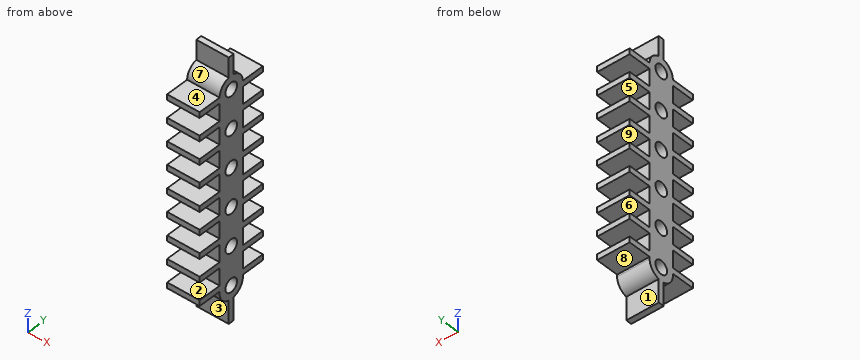
```python
from build123d import *

# Parameters (mm, degrees)
SKETCH1_R           = 17.5
BOSS_EXTRUDE1_DEPTH = 85


with BuildPart() as part:
    # Sketch1 → Boss-Extrude1 (new body)
    with BuildSketch(Plane(origin=(0, 0, 0), x_dir=(0, 0, -1), z_dir=(1, 0, 0))):
        with BuildLine():
            Line((-250.081967213, 35), (-205.081967213, 35))
            Line((-205.081967213, 35), (-205.081967213, 95))
            Line((-205.081967213, 95), (-190.081967213, 95))
            Line((-190.081967213, 95), (-190.081967213, 35))
            Line((-190.081967213, 35), (-185.081967213, 35))
            Line((-185.081967213, 35), (-145.081967213, 35))
            Line((-145.081967213, 35), (-145.081967213, 95))
            Line((-145.081967213, 95), (-130.081967213, 95))
            Line((-130.081967213, 95), (-130.081967213, 35))
            Line((-130.081967213, 35), (-85.081967213, 35))
            Line((-85.081967213, 35), (-85.081967213, 95))
            Line((-85.081967213, 95), (-70.081967213, 95))
            Line((-70.081967213, 95), (-70.081967213, 35))
            Line((-70.081967213, 35), (-25.081967213, 35))
            Line((-25.081967213, 35), (-25.081967213, 95))
            Line((-25.081967213, 95), (-10.081967213, 95))
            Line((-10.081967213, 95), (-10.081967213, 35))
            Line((-10.081967213, 35), (34.918032787, 35))
            Line((34.918032787, 35), (34.918032787, 95))
            Line((34.918032787, 95), (49.918032787, 95))
            Line((49.918032787, 95), (49.918032787, 35))
            Line((49.918032787, 35), (94.918032787, 35))
            Line((94.918032787, 35), (94.918032787, 95))
            Line((94.918032787, 95), (109.918032787, 95))
            Line((109.918032787, 95), (109.918032787, 35))
            Line((109.918032787, 35), (154.918032787, 35))
            Line((154.918032787, 35), (154.918032787, 95))
            Line((154.918032787, 95), (169.918032787, 95))
            Line((169.918032787, 95), (169.918032787, 35))
            Line((169.918032787, 35), (214.918032787, 35))
            Line((214.918032787, 35), (214.918032787, 95))
            Line((214.918032787, 95), (229.918032787, 95))
            Line((229.918032787, 95), (229.918032787, 35))
            Line((229.918032787, 35), (235.374517149, 35))
            ThreePointArc((235.374517149, 35), (257.311928117, 27.271780287), (269.561502977, 7.5))
            Line((269.561502977, 7.5), (329.561502977, 7.5))
            Line((329.561502977, 7.5), (329.561502977, -7.5))
            Line((329.561502977, -7.5), (269.561502977, -7.5))
            ThreePointArc((269.561502977, -7.5), (257.311928117, -27.271780287), (235.374517149, -35))
            Line((235.374517149, -35), (229.918032787, -35))
            Line((229.918032787, -35), (229.918032787, -95))
            Line((229.918032787, -95), (214.918032787, -95))
            Line((214.918032787, -95), (214.918032787, -35))
            Line((214.918032787, -35), (169.918032787, -35))
            Line((169.918032787, -35), (169.918032787, -95))
            Line((169.918032787, -95), (154.918032787, -95))
            Line((154.918032787, -95), (154.918032787, -35))
            Line((154.918032787, -35), (109.918032787, -35))
            Line((109.918032787, -35), (109.918032787, -95))
            Line((109.918032787, -95), (94.918032787, -95))
            Line((94.918032787, -95), (94.918032787, -35))
            Line((94.918032787, -35), (49.918032787, -35))
            Line((49.918032787, -35), (49.918032787, -95))
            Line((49.918032787, -95), (34.918032787, -95))
            Line((34.918032787, -95), (34.918032787, -35))
            Line((34.918032787, -35), (-10.081967213, -35))
            Line((-10.081967213, -35), (-10.081967213, -95))
            Line((-10.081967213, -95), (-25.081967213, -95))
            Line((-25.081967213, -95), (-25.081967213, -35))
            Line((-25.081967213, -35), (-70.081967213, -35))
            Line((-70.081967213, -35), (-70.081967213, -95))
            Line((-70.081967213, -95), (-85.081967213, -95))
            Line((-85.081967213, -95), (-85.081967213, -35))
            Line((-85.081967213, -35), (-130.081967213, -35))
            Line((-130.081967213, -35), (-130.081967213, -95))
            Line((-130.081967213, -95), (-145.081967213, -95))
            Line((-145.081967213, -95), (-145.081967213, -35))
            Line((-145.081967213, -35), (-190.081967213, -35))
            Line((-190.081967213, -35), (-190.081967213, -95))
            Line((-190.081967213, -95), (-205.081967213, -95))
            Line((-205.081967213, -95), (-205.081967213, -35))
            Line((-205.081967213, -35), (-250.081967213, -35))
            Line((-250.081967213, -35), (-250.081967213, -95))
            Line((-250.081967213, -95), (-265.081967213, -95))
            Line((-265.081967213, -95), (-265.081967213, -35))
            ThreePointArc((-265.081967213, -35), (-286.793224125, -27.156121863), (-298.898676377, -7.5))
            Line((-298.898676377, -7.5), (-350.428459553, -7.5))
            Line((-350.428459553, -7.5), (-350.428459553, 7.5))
            Line((-350.428459553, 7.5), (-298.898676377, 7.5))
            ThreePointArc((-298.898676377, 7.5), (-286.793224125, 27.156121863), (-265.081967213, 35))
            Line((-265.081967213, 35), (-265.081967213, 95))
            Line((-265.081967213, 95), (-250.081967213, 95))
            Line((-250.081967213, 95), (-250.081967213, 35))
        make_face()
        with Locations((-264.709663373, 0)):
            Circle(SKETCH1_R, mode=Mode.SUBTRACT)
        with Locations((-164.709663373, 0)):
            Circle(SKETCH1_R, mode=Mode.SUBTRACT)
        with Locations((-64.709663373, 0)):
            Circle(SKETCH1_R, mode=Mode.SUBTRACT)
        with Locations((35.290336627, 0)):
            Circle(SKETCH1_R, mode=Mode.SUBTRACT)
        with Locations((135.290336627, 0)):
            Circle(SKETCH1_R, mode=Mode.SUBTRACT)
        with Locations((235.290336627, 0)):
            Circle(SKETCH1_R, mode=Mode.SUBTRACT)
    extrude(amount=BOSS_EXTRUDE1_DEPTH)


solid = part.part
```
Source: CAD feature listing. Evaluate the final solid. Frame: model axes, mm. Face numbers are marked on the shaded views. A direction names the side the tool comes from. Coordinates: 2 decimals unless noted, no trailing zeros. Write each loop counter-clockwise with the first axis right and the second up, starting at its lowest first coordinate (ties: lowest second). Pieces come first, ordered by that corner, then holes. Notation, with made-up numbers: (80, -11) -> (114, -11) arc R14 cw to (114, 5) -> close; hole circle Ø8 at (10, 37). An arc over 180 degrees is marked (long way). Return JSON: item names as keys, results as strings. Group by question number.
1) Mould query, pull axis Z, two halves, no side actions, for the marked faces 6, 7, 8 and 9. Classes: +Z half, -Z half, draft (parallel to the pull), parting line (faces both ways), or undercut.
2) Section query A-A, the plane y = 0. Return loops of the section in (x, z).
3) Contact query for flat-ended pins moving along their axis: P1, Ø3, axis at y = 65, z = 127.5, coming from the +X side; P2, Ø4, axis at x = 56.5, z = 177, coming from the +Y side; P3, Ø3, axis at x = 56.5, y = 46, coming from the +Z side; P4, Ø1, axis at x = 36.5, z = -125.5, coming from the -Y side. Output: stop coordinate, or through.
4) Section query C-C, the plane x = 61. State how many separate pieces and enclosed holes the cut face has, plus the area to 3 significant figures.
5) Section query B-B, the plane z = 172. Return loops of the section in (x, y).
6) Set-up query: the marked faces 1, 2, 3, 4 and 5. Return all of +Z, -Z, +X, -X, +Y, -Y with unobstructed straight access to the full face (end or side cutting, diameter ignored); none if empty.
7) Ray query, line 1 along Y through (x, z) = (74, 126); line 2 along Y through (x, z) = (69.5, 251); line 3 along Y through (x, z) = (57.5, 68.5). Return the intervals inside material, ascending.
From the geometry:
{
 "1": {"face 6": "undercut", "face 7": "+Z half", "face 8": "-Z half", "face 9": "undercut"},
 "2": {"outline": "(0, -329.56) -> (85, -329.56) -> (85, -252.79) -> (0, -252.79) -> close; (0, -217.79) -> (85, -217.79) -> (85, -152.79) -> (0, -152.79) -> close; (0, -117.79) -> (85, -117.79) -> (85, -52.79) -> (0, -52.79) -> close; (0, -17.79) -> (85, -17.79) -> (85, 47.21) -> (0, 47.21) -> close; (0, 82.21) -> (85, 82.21) -> (85, 147.21) -> (0, 147.21) -> close; (0, 182.21) -> (85, 182.21) -> (85, 247.21) -> (0, 247.21) -> close; (0, 282.21) -> (85, 282.21) -> (85, 350.43) -> (0, 350.43) -> close"},
 "3": {"P1": "through", "P2": "y = 35", "P3": "z = 265.08", "P4": "y = -35"},
 "4": {"separate pieces": "1", "enclosed holes": "6", "area": "50,900 mm²"},
 "5": {"outline": "(0, -35) -> (85, -35) -> (85, -15.91) -> (0, -15.91) -> close; (0, 15.91) -> (85, 15.91) -> (85, 35) -> (0, 35) -> close"},
 "6": {"face 1": "-Z, +X, -X, +Y", "face 2": "+X, -X, -Y", "face 3": "-Z, +X, -X, -Y", "face 4": "+Z, +X, -X, -Y", "face 5": "+X, -X, +Y"},
 "7": {"line 1": "-35 to 35", "line 2": "-95 to -10.88, 10.88 to 95", "line 3": "-35 to -17.08, 17.08 to 35"}
}
